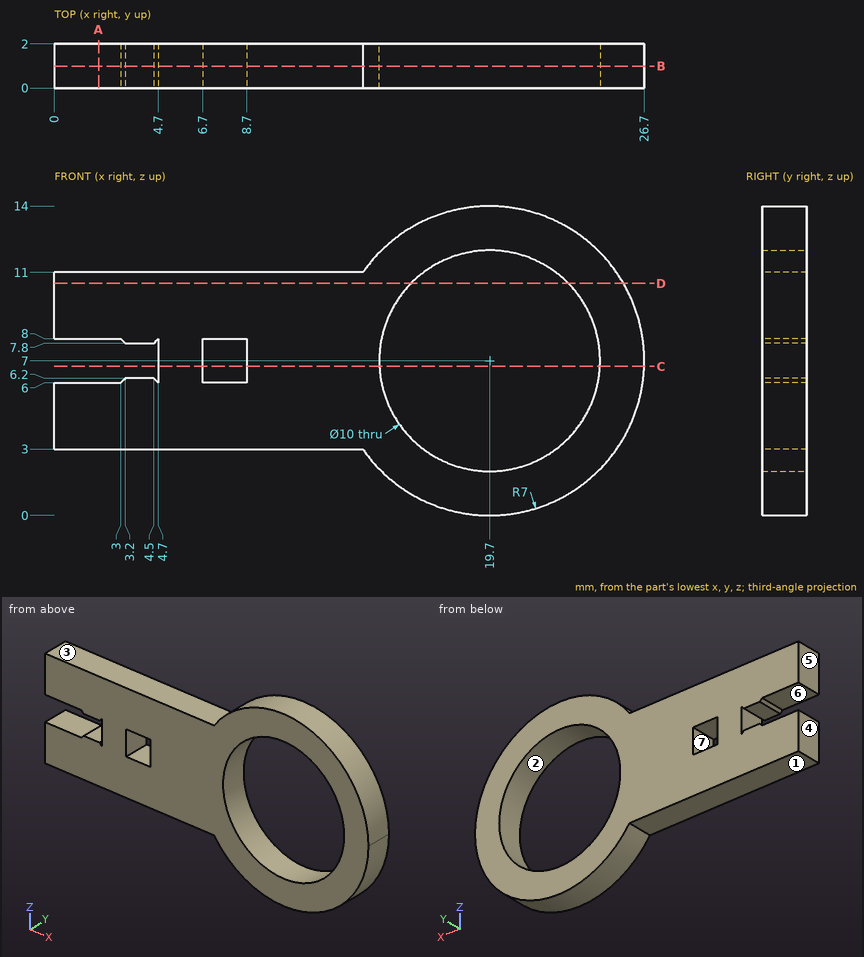
Source: three-view drawing plus pictorial views. Frame: mm from the lowest corner of the part. A direction names the side the tool comes from. Coordinates: 2 decimals unless noted, no trailing zeros. Loops run counter-clockwise (first coordinate to the right, second up) from the corner with the lowest first, then second, coordinate; pieces in that order, holes last. Notation, with made-up numbers: M -35.5,52.25 L -8.5,52.25 A4 ccw -8.5,57.25 Z; hole C -33,-22 d1. An arc over 180 degrees is marked long. Use CSV: the item, a comma, the result in double quotes.
(1) Draft query along Z for the marked faces 1, 2, 3 and 4. Return one class per face: pulls with the +Z half, pulls with the -Z half, needs draft (parallel to the pull), parting line crosses it, or undercut.
Answers follow:
face 1,"pulls with the -Z half"
face 2,"undercut"
face 3,"pulls with the +Z half"
face 4,"needs draft"
(2) Reachability of the marked faces 5, 6 and 7 from +Z, -Z, +X, -X, +Y, -Y: full face, straight path, thin tool, end or side. Return the list, or none.
Answers follow:
face 5,"+Z, -Z, -X, +Y, -Y"
face 6,"-X, +Y, -Y"
face 7,"+Y, -Y"
(3) Cut plane C-C on z = 6.75. Return loops of the section in (x, y), and give its area (3 significant figures).
Answers follow:
outline,"M 4.7,0 L 6.7,0 L 6.7,2 L 4.7,2 Z; M 8.7,0 L 14.71,0 L 14.71,2 L 8.7,2 Z; M 24.69,0 L 26.7,0 L 26.7,2 L 24.69,2 Z"
area,"20.0 mm²"
(4) Cut plane B-B on y = 1. Return loops of the section in (x, z).
Answers follow:
outline,"M 0,3 L 13.96,3 A7 ccw long 13.96,11 L 0,11 L 0,8 L 3,8 L 3.2,7.8 L 4.5,7.8 L 4.7,8 L 4.7,6 L 4.5,6.2 L 3.2,6.2 L 3,6 L 0,6 Z; hole M 6.7,6 L 8.7,6 L 8.7,8 L 6.7,8 Z; hole C 19.7,7 d10"
(5) Cut plane A-A on x = 2. Return loops of the section in (y, z), and give its area (3 significant figures).
Answers follow:
outline,"M 0,3 L 2,3 L 2,6 L 0,6 Z; M 0,8 L 2,8 L 2,11 L 0,11 Z"
area,"12.0 mm²"
(6) Line query: line 1 (Z direction, x = 7.25, y = 1.85); line 2 (Z direction, x = 19.7, y = 1.15); line 3 (X direction, y = 1.55, z = 9.25). Output: solid intervals per line, ascending. Write a range as [from, to].
Answers follow:
line 1,"[3, 6], [8, 11]"
line 2,"[0, 2], [12, 14]"
line 3,"[0, 15.23], [24.17, 26.33]"
(7) Contact query for flat-ended pins moving along their axis: pin 1 (1 mm diameter, centred on x = 1, y = 1, fed in from -Z); pin 2 (1 mm diameter, centred on x = 10, y = 0.5, fed in from +Z); pin 3 (1.5 mm diameter, centred on x = 5, z = 12, fed in from +Y). Output: stop coordinate, or through.
Answers follow:
pin 1,"z = 3"
pin 2,"z = 11"
pin 3,"through"
(8) Cut plane D-D on z = 10.5. Return loops of the section in (x, y), and give its area (3 significant figures).
Answers follow:
outline,"M 0,0 L 16.13,0 L 16.13,2 L 0,2 Z; M 23.27,0 L 25.76,0 L 25.76,2 L 23.27,2 Z"
area,"37.2 mm²"
